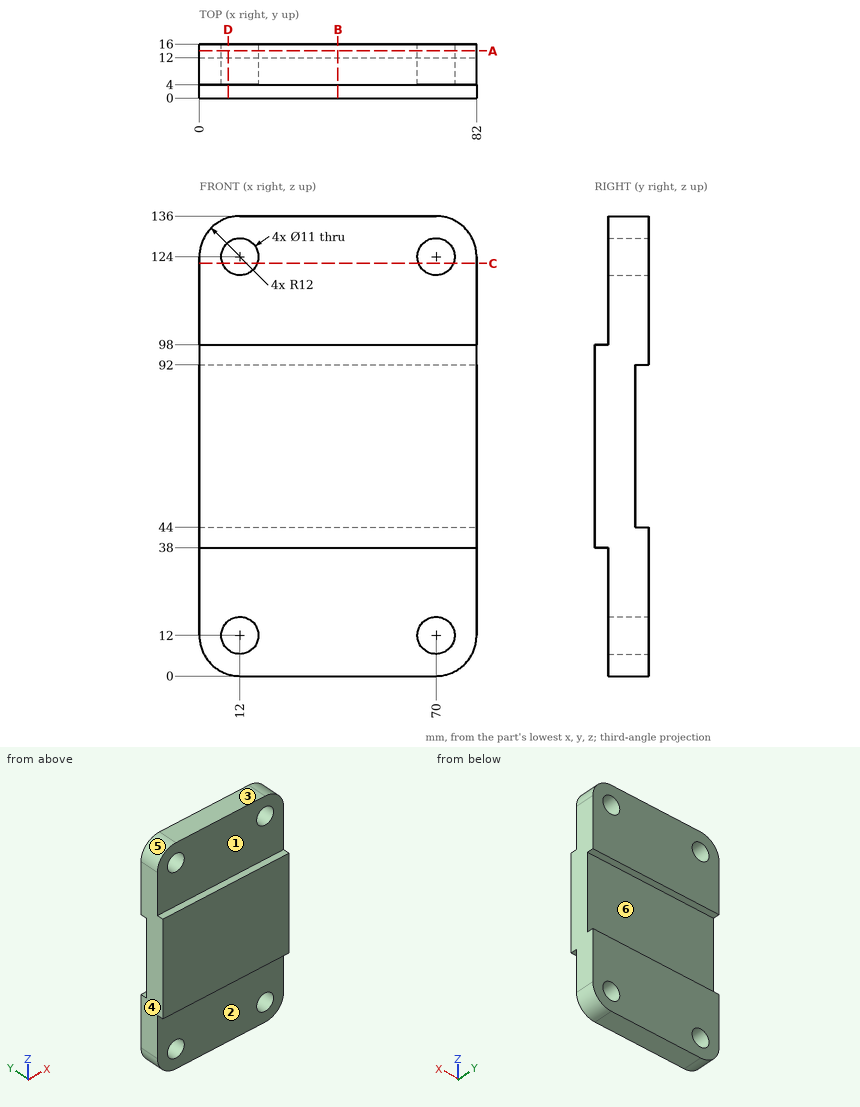
Study the drawing (mm; zero at the part's minimum x, y, z) and answer. A direction names the side the tool comes from. Coordinates: 2 decimals unless noted, no trailing zeros. Write each loop counter-clockwise with the first axis right and the second up, starting at its lowest first coordinate (ties: lowest second). Pieces come first, ordered by that corner, then holes. Notation, with made-up numbers: (18.25, 11) - (38.25, 11) arc R21 ccw to (38.25, 40) - close; hole circle Ø8 at (77.5, 2). An arc over 180 degrees is marked (long way). Put each result on its own line as item: value.
1. Flat-ended cylindrical pins translate along their axes: pin 1 Ø6.5 at (x, z) = (12, 12) entering from -Y; pin 2 Ø3 at (x, y) = (28.5, 1) entering from +Z; pin 3 Ø24 at (x, z) = (34, 73) entering from +Y; pin 4 Ø1.2 at (x, y) = (27.5, 1) entering from -Z. Find the tip coordinate at first contact, or state that the pin passes through.
Answer sheet:
pin 1: passes through
pin 2: stops at z = 98
pin 3: stops at y = 12
pin 4: stops at z = 38
2. The part is cut by section C-C on z = 122. Give the vertices of the cut face in (x, y), plus the area to 3 significant figures.
Answer sheet:
outline: (0, 4) - (6.88, 4) - (6.88, 16) - (0, 16) - close; (17.12, 4) - (64.88, 4) - (64.88, 16) - (17.12, 16) - close; (75.12, 4) - (82, 4) - (82, 16) - (75.12, 16) - close
area: 738 mm^2
3. A tool of negligible diameter and unlimited length cuts with its end or side. For the marked faces 1, 2 and 3, from which of +Z, -Z, +X, -X, +Y, -Y can it reach the whole face along a straight path? Write none if from no direction.
Answer sheet:
face 1: +Z, +X, -X, -Y
face 2: -Z, +X, -X, -Y
face 3: +Z, +X, -X, +Y, -Y
4. Determine the mould class of the marked faces 4, 5 and 6 for opening direction Z: pulls with the +Z half, pulls with the -Z half, needs draft (parallel to the pull), parting line crosses it, or undercut.
Answer sheet:
face 4: needs draft
face 5: pulls with the +Z half
face 6: undercut
5. The part is cut by section D-D on x = 8.5. Give the vertices of the cut face in (y, z), plus the area to 3 significant figures.
Answer sheet:
outline: (0, 38) - (4, 38) - (4, 16.24) - (16, 16.24) - (16, 44) - (12, 44) - (12, 92) - (16, 92) - (16, 119.76) - (4, 119.76) - (4, 98) - (0, 98) - close; (4, 0.52) - (16, 0.52) - (16, 7.76) - (4, 7.76) - close; (4, 128.24) - (16, 128.24) - (16, 135.48) - (4, 135.48) - close
area: 1,460 mm^2
6. Find the intervals of material crossed by line 1 along X through (y, z) = (7, 124); line 2 along Z through (x, y) = (12, 12.25); line 3 along Z through (x, y) = (12, 6.75), in increasing order. Write a range as from..to.
Answer sheet:
line 1: x = 0..6.5, 17.5..64.5, 75.5..82
line 2: z = 0..6.5, 17.5..44, 92..118.5, 129.5..136
line 3: z = 0..6.5, 17.5..118.5, 129.5..136
7. The part is cut by section B-B on x = 41. Give the vertices of the cut face in (y, z).
Answer sheet:
outline: (0, 38) - (4, 38) - (4, 0) - (16, 0) - (16, 44) - (12, 44) - (12, 92) - (16, 92) - (16, 136) - (4, 136) - (4, 98) - (0, 98) - close
8. The part is cut by section A-A on y = 14. Give the vertices of the cut face in (x, z), plus the area to 3 significant figures.
Answer sheet:
outline: (0, 12) arc R12 ccw to (12, 0) - (70, 0) arc R12 ccw to (82, 12) - (82, 44) - (0, 44) - close; (0, 92) - (82, 92) - (82, 124) arc R12 ccw to (70, 136) - (12, 136) arc R12 ccw to (0, 124) - close; hole circle Ø11 at (12, 12); hole circle Ø11 at (12, 124); hole circle Ø11 at (70, 12); hole circle Ø11 at (70, 124)
area: 6,710 mm^2
